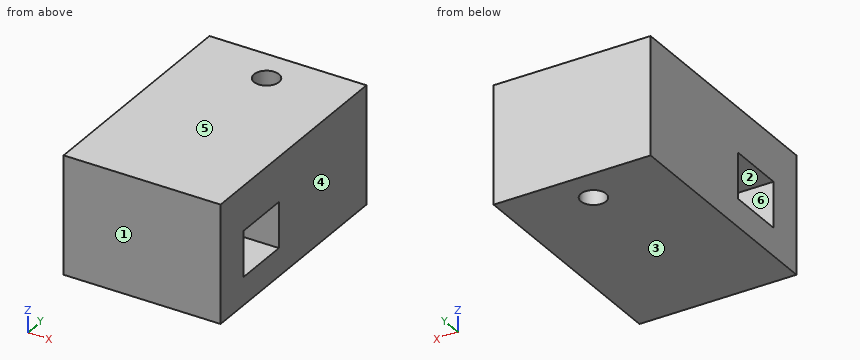
from build123d import *

# Parameters (mm, degrees)
F0_W     = 25.4
F0_H     = 38.1
F1_DEPTH = 19.05
F2_R     = 2.032
F3_DEPTH = 25.4
F4_W     = 9.271
F4_H     = 7.366
F5_DEPTH = 25.4


with BuildPart() as f1:
    # F0 (on Top) → F1 (new body)
    with BuildSketch(Plane.XY):
        with Locations((0, -6.35)):
            Rectangle(F0_W, F0_H)
    extrude(amount=F1_DEPTH)

    # F2 (on face) → F3 (cut)
    with BuildSketch(Plane.XY.offset(19.05)):
        with Locations((0, 7.112)):
            Circle(F2_R)
    extrude(amount=-F3_DEPTH, mode=Mode.SUBTRACT)

    # F4 (on face) → F5 (cut)
    with BuildSketch(Plane.YZ.offset(12.7)):
        with Locations((-14.7955, 8.179266)):
            Rectangle(F4_W, F4_H)
    extrude(amount=-F5_DEPTH, mode=Mode.SUBTRACT)


solid = f1.part
Geometry check sheet. Reference: the model listing, model coordinates, mm. Face numbers are marked on the shaded views. A direction names the side the tool comes from. Round coordinates to 2 decimals unless told otherwise and drop trailing zeros. Loops run counter-clockwise (first coordinate to the right, second up) from the corner with the lowest first, then second, coordinate; pieces in that order, holes last.
Item 1: Access from +Z, -Z, +X, -X, +Y, -Y to the whole of each face (thin tool, end or side, straight path). Record for the marked faces 1 and 2.
Item 2: Gauge pin test, flat end, axial feed: pin 1 (7.5 mm diameter, centred on x = 5, y = -16, fed in from -Z). Record the tip position at first contact, or that the pin passes through.
Item 3: Cross-section at D-D on x = 8.25. Record the boundary of the cut face in (y, z), then the cut area to 3 significant figures.
Item 4: Cross-section at B-B on y = -16.5. Record the boundary of the cut face in (x, z), then the cut area to 3 significant figures.
Item 5: Cross-section at C-C on z = 7. Record the boundary of the cut face in (x, y).
Item 6: Thickness scan on line 1 (Y direction, x = 0, z = 6); line 2 (Y direction, x = 4, z = 7.75); line 3 (Z direction, x = 7, y = -16). Record the ranges inside material, lowest first.
Item 7: Mould release check, pull along Z, two halves, no side actions. Record for the marked faces 3, 4, 5 and 6: pulls with the +Z half, pulls with the -Z half, needs draft (parallel to the pull), parting line crosses it, or undercut.
Item 8: Cross-section at A-A on x = 0. Record the boundary of the cut face in (y, z).
Answer sheet:
1. face 1: +Z, -Z, +X, -X, -Y
1. face 2: +X, -X
2. pin 1: stops at z = 0
3. outline: (-25.4, 0) - (12.7, 0) - (12.7, 19.05) - (-25.4, 19.05) - close; hole (-19.43, 4.5) - (-10.16, 4.5) - (-10.16, 11.86) - (-19.43, 11.86) - close
3. area: 658 mm2
4. outline: (-12.7, 0) - (12.7, 0) - (12.7, 4.5) - (-12.7, 4.5) - close; (-12.7, 11.86) - (12.7, 11.86) - (12.7, 19.05) - (-12.7, 19.05) - close
4. area: 297 mm2
5. outline: (-12.7, -25.4) - (12.7, -25.4) - (12.7, -19.43) - (-12.7, -19.43) - close; (-12.7, -10.16) - (12.7, -10.16) - (12.7, 12.7) - (-12.7, 12.7) - close; hole circle Ø4.06 at (0, 7.11)
6. line 1: y = -25.4 to -19.43, -10.16 to 5.08, 9.14 to 12.7
6. line 2: y = -25.4 to -19.43, -10.16 to 12.7
6. line 3: z = 0 to 4.5, 11.86 to 19.05
7. face 3: pulls with the -Z half
7. face 4: needs draft
7. face 5: pulls with the +Z half
7. face 6: undercut
8. outline: (-25.4, 0) - (5.08, 0) - (5.08, 19.05) - (-25.4, 19.05) - close; (9.14, 0) - (12.7, 0) - (12.7, 19.05) - (9.14, 19.05) - close; hole (-19.43, 4.5) - (-10.16, 4.5) - (-10.16, 11.86) - (-19.43, 11.86) - close
